Could you check a few things on this model? Use its own coordinates, in mm. A direction names the side the tool comes from. Give positions to 0.01 mm unless a question says otherwise; leave off trailing zeros. Loops run counter-clockwise (first coordinate to the right, second up) from the corner with the lowest first, then second, coordinate; pieces in that order, holes last. Notation, with made-up numbers: (-2.5, 61.5) -> (3.5, 61.5) arc R17 cw to (3.5, 81.5) -> close; hole circle Ø1 at (67.25, 0.25). An arc over 180 degrees is marked (long way). Write item = value, one per line. Start each with the question number.
1) I want a section at A-A (x = 4.5). List the corners of the cut face in (y, z) for me.
2) I want a section at B-B (z = 3.75). List the corners of the cut face in (x, y) for me, and give its area (3 significant figures).
3) I want a section at D-D (z = 0). List the corners of the cut face in (x, y) for me, and give its area (3 significant figures).
4) If we mould it in two halves opening along Y, with no side actions, what happens to faces 1 (the face through (0, 0, -7.5)), 2 (the face through (-1.63, -7.32, 0.11))? For each: +Y half, -Y half, draft (parallel to the pull), parting line (faces both ways), or undercut.
5) I'm going to push flat-ended pins straight in: pin 1 Ø6 at (x, z) = (3.5, 5) entering from +Y; pin 2 Ø4 at (y, z) = (36.5, -2.5) entering from -X; pin 3 Ø3 at (y, z) = (29.5, 0.5) entering from -X. Where does each tip first touch, or does it pass through?
6) On a 3-axis mill with a long thin cutter (end or side, diameter ignored), from which of +Z, -Z, +X, -X, +Y, -Y can I reach the whole of each face in a straight line? I mean faces 3 (the face through (2, 39, 0)), 4 (the face through (0, 78, -7.5)). Say none if no direction works.
7) I want a section at C-C (y = 12.5). List the corners of the cut face in (x, z) for me.
8) I need wall thicknesses on probe 1 along Y at (x, z) = (0.5, -4); probe 2 along Y at (x, z) = (-5.75, 7.25); probe 3 along X at (y, z) = (81.5, 3.25). Which ranges of each line are inside material? Lowest first, please. Write a range as from..to.
from build123d import *

# Parameters (mm, degrees)
SKETCH2_R           = 7.5
BOSS_EXTRUDE1_DEPTH = 7.5
SKETCH4_R           = 2
BOSS_EXTRUDE2_DEPTH = 78
LPATTERN1_COUNT     = 2
LPATTERN1_PITCH     = 78


with BuildPart() as part:
    # Sketch2 → Boss-Extrude1 (new, symmetric)
    with BuildSketch(Plane.XY):
        Circle(SKETCH2_R)
    boss_extrude1 = extrude(amount=BOSS_EXTRUDE1_DEPTH, both=True)

    # Sketch4 → Boss-Extrude2 (add)
    with BuildSketch(Plane(origin=(0, 0, 0), x_dir=(1, 0, 0), z_dir=(0, 1, 0))):
        with Locations(Location((0, 0, 0), (0, 0, 90))):
            Circle(SKETCH4_R)
    extrude(amount=BOSS_EXTRUDE2_DEPTH)

    # LPattern1: Boss-Extrude1 ×2
    with Locations(*[(0, i * LPATTERN1_PITCH, 0) for i in range(1, LPATTERN1_COUNT)]):
        add(boss_extrude1)


solid = part.part
Answer list:
q1.outline = (-6, -7.5) -> (6, -7.5) -> (6, 7.5) -> (-6, 7.5) -> close; (72, -7.5) -> (84, -7.5) -> (84, 7.5) -> (72, 7.5) -> close
q2.outline = circle Ø15 at (0, 0); circle Ø15 at (0, 78)
q2.area = 353 mm^2
q3.outline = (-2, 7.23) arc R7.5 ccw (long way) to (2, 7.23) -> (2, 70.77) arc R7.5 ccw (long way) to (-2, 70.77) -> close
q3.area = 606 mm^2
q4.face_1 = draft
q4.face_2 = undercut
q5.pin_1 = 85.48
q5.pin_2 = -1.94
q5.pin_3 = -2
q6.face_3 = none
q6.face_4 = -Z, +X, -X, +Y, -Y
q7.outline = circle Ø4 at (0, 0)
q8.probe_1 = -7.48..7.48, 70.52..85.48
q8.probe_2 = -4.82..4.82, 73.18..82.82
q8.probe_3 = -6.63..6.63
